Design review of the part built by this model. Coordinates are the model's own, in mm. A direction names the side the tool comes from. Coordinates: 2 decimals unless noted, no trailing zeros. Write each loop counter-clockwise with the first axis right and the second up, starting at its lowest first coordinate (ties: lowest second). Pieces come first, ordered by that corner, then holes. Notation, with made-up numbers: (-10, -40) - (26, -40) arc R16 cw to (26, -11) - close; hole circle Ø6 at (3.25, 4). An arc over 180 degrees is marked (long way). One line per item, written item: value.
from build123d import *

# Parameters (mm, degrees)
SKETCH1_W           = 80
SKETCH1_H           = 120
BOSS_EXTRUDE1_DEPTH = 2
SKETCH2_R           = 1.5
CUT_EXTRUDE1_DEPTH  = 145.235917857
CUT_EXTRUDE2_DEPTH  = 145.235917857
FILLET1_R           = 2


with BuildPart() as part:
    # Sketch1 → Boss-Extrude1 (new body)
    with BuildSketch(Plane(origin=(0, 0, 0), x_dir=(1, 0, 0), z_dir=(0, 1, 0))):
        with Locations((40, 60)):
            Rectangle(SKETCH1_W, SKETCH1_H)
    extrude(amount=BOSS_EXTRUDE1_DEPTH)

    # Sketch2 → Cut-Extrude1 (cut, through all)
    with BuildSketch(Plane(origin=(0, 2, 0), x_dir=(1, 0, 0), z_dir=(0, 1, 0))):
        with Locations(Location((2.75, 115, 0), (0, 0, 270))):
            Circle(SKETCH2_R)
        with Locations(Location((77.25, 115, 0), (0, 0, 90))):
            Circle(SKETCH2_R)
        with Locations(Location((77.25, 5, 0), (0, 0, 270))):
            Circle(SKETCH2_R)
        with Locations(Location((2.75, 21.35, 0), (0, 0, 270))):
            Circle(SKETCH2_R)
    extrude(amount=-CUT_EXTRUDE1_DEPTH, mode=Mode.SUBTRACT)

    # Sketch3 → Cut-Extrude2 (cut, through all)
    with BuildSketch(Plane(origin=(0, 2, 0), x_dir=(1, 0, 0), z_dir=(0, 1, 0))):
        with BuildLine():
            Line((2.75, 128.5), (77.25, 128.5))
            ThreePointArc((77.25, 128.5), (69.809659383, 126.264605253), (64.833333333, 120.298715777))
            ThreePointArc((64.833333333, 120.298715777), (40, 103.896147332), (15.166666667, 120.298715777))
            ThreePointArc((15.166666667, 120.298715777), (10.190340617, 126.264605253), (2.75, 128.5))
        make_face()
        with BuildLine():
            Line((-10.75, 115), (-10.75, 21.35))
            ThreePointArc((-10.75, 21.35), (-7.967575093, 29.558750461), (-0.767246795, 34.383762887))
            ThreePointArc((-0.767246795, 34.383762887), (25.113965218, 68.175), (-0.767246795, 101.966237113))
            ThreePointArc((-0.767246795, 101.966237113), (-7.967575093, 106.791249539), (-10.75, 115))
        make_face()
        with BuildLine():
            Line((-10.75, 7.85), (-10.75, -8.5))
            Line((-10.75, -8.5), (77.25, -8.5))
            ThreePointArc((77.25, -8.5), (69.997734791, -6.386599551), (65.016127441, -0.708096198))
            ThreePointArc((65.016127441, -0.708096198), (41.147259356, 18.402573211), (11.469252441, 11.043466302))
            ThreePointArc((11.469252441, 11.043466302), (7.392832922, 8.673482242), (2.75, 7.85))
            Line((2.75, 7.85), (-10.75, 7.85))
        make_face()
        with BuildLine():
            Line((90.75, 5), (90.75, 115))
            ThreePointArc((90.75, 115), (87.723180033, 106.481637481), (80, 101.783060112))
            ThreePointArc((80, 101.783060112), (46.015741918, 60), (80, 18.216939888))
            ThreePointArc((80, 18.216939888), (87.723180033, 13.518362519), (90.75, 5))
        make_face()
    extrude(amount=-CUT_EXTRUDE2_DEPTH, mode=Mode.SUBTRACT)

    # Fillet1
    fillet1_edges = [part.edges().sort_by_distance(p)[0] for p in [
        (0, 1, -101.749786914),
        (0, 1, -34.600213086),
        (64.675872748, 1, 0),
        (0, 1, -7.85),
        (80, 1, -18.216939888),
        (80, 1, -101.783060112),
        (0, 1, -120),
        (80, 1, -120),
        (64.703723876, 1, -120),
        (80, 1, 0),
        (15.296276124, 1, -120),
    ]]
    fillet(fillet1_edges, radius=FILLET1_R)


solid = part.part
1. For faces 4 (the face through (2.8, 1, -116.5)), 5 (the face through (7.46, 1.01, -8.7)), list the 3-axis set-ups (+Z, -Z, +X, -X, +Y, -Y) from which the entire face can be reached by the end or side of a thin tool; tool diameter is ignored.
Answer block:
face 4: +Y, -Y
face 5: +Z, +Y, -Y
2. Insertion check: pin 1 Ø8 at (x, z) = (48, -81.5) entering from -Y; pin 2 Ø1 at (x, y) = (54.5, 1.5) entering from -Z. Each pin has a flat end and moves straight along its axis. Give the tip position at first contact, or say it passes through.
Answer block:
pin 1: stops at y = 0
pin 2: stops at z = -108.45
3. Consider section C-C, the plane z = -21.35. Write out the cut boundary in (x, y).
Answer block:
outline: (0, 0) - (1.25, 0) - (1.25, 2) - (0, 2) - close; (4.25, 0) - (70.59, 0) - (70.59, 2) - (4.25, 2) - close
4. Consider section A-A, the plane y = 0.6. Write out the cut boundary in (x, z) (3 decimals).
Answer block:
outline: (0, -118) arc R2 ccw to (2, -120) - (14.025, -120) arc R2 ccw to (15.817, -118.889) arc R27 cw to (64.183, -118.889) arc R2 ccw to (65.975, -120) - (78, -120) arc R2 ccw to (80, -118) - (80, -103.379) arc R2 ccw to (78.479, -101.437) arc R42.678 cw to (78.479, -18.563) arc R2 ccw to (80, -16.621) - (80, -2) arc R2 ccw to (78, 0) - (65.894, 0) arc R2 ccw to (64.133, -1.052) arc R34.5 cw to (11.469, -11.043) arc R13.5 ccw to (2.75, -7.85) - (2, -7.85) arc R2 ccw to (0, -9.85) - (0, -33.136) arc R2 ccw to (1.358, -35.03) arc R35 cw to (1.358, -101.32) arc R2 ccw to (0, -103.214) - close; hole circle Ø3 at (2.75, -115); hole circle Ø3 at (2.75, -21.35); hole circle Ø3 at (77.25, -115); hole circle Ø3 at (77.25, -5)
5. Wall thickness on line 1 along X through (y, z) = (1, -115); line 2 along X through (y, z) = (1.1, -21.35); line 3 along Z through (x, y) = (77.25, 1.35): over which ranges is each line inside the solid? List them lowest first.
Answer block:
line 1: x = 0 to 1.25, 4.25 to 18.18, 61.82 to 75.75, 78.75 to 80
line 2: x = 0 to 1.25, 4.25 to 70.59
line 3: z = -120 to -116.5, -113.5 to -101.12, -18.88 to -6.5, -3.5 to 0
6. Mouldability with a two-part tool opening along X and no side actions: class faces 1 (the face through (25.11, 1.01, -67.57)), 2 (the face through (40.4, 1, -103.9)), 3 (the face through (39, 2, -61)) as released by +X, released by -X, zero draft, split by the parting line, or undercut.
Answer block:
face 1: released by -X
face 2: undercut
face 3: zero draft
7. Consider section D-D, the plane z = -115. Write out the cut boundary in (x, y).
Answer block:
outline: (0, 0) - (1.25, 0) - (1.25, 2) - (0, 2) - close; (4.25, 0) - (18.18, 0) - (18.18, 2) - (4.25, 2) - close; (61.82, 0) - (75.75, 0) - (75.75, 2) - (61.82, 2) - close; (78.75, 0) - (80, 0) - (80, 2) - (78.75, 2) - close
8. Consider section B-B, the plane x = 51.5. Write out the cut boundary in (y, z).
Answer block:
outline: (0, -106.47) - (2, -106.47) - (2, -80.93) - (0, -80.93) - close; (0, -39.07) - (2, -39.07) - (2, -14.29) - (0, -14.29) - close
